from build123d import *

# Parameters (mm, degrees)
CROQUIS1_R              = 5.5
SALIENTE_EXTRUIR1_DEPTH = 10
CROQUIS3_W              = 5.5
CROQUIS3_H              = 15.5
SALIENTE_EXTRUIR2_DEPTH = 3


with BuildPart() as part:
    # Croquis1 → Saliente-Extruir1 (new body)
    with BuildSketch(Plane(origin=(0, 0, 0), x_dir=(1, 0, 0), z_dir=(0, 1, 0))):
        with Locations(Location((-6.881511077, -6.29378807, 0), (0, 0, 270))):
            Circle(CROQUIS1_R)
    extrude(amount=SALIENTE_EXTRUIR1_DEPTH)

    # Croquis3 → Saliente-Extruir2 (add)
    with BuildSketch(Plane(origin=(0, 0, 0), x_dir=(1, 0, 0), z_dir=(0, 1, 0))):
        with Locations((-6.881511077, -6.29378807)):
            Rectangle(CROQUIS3_W, CROQUIS3_H)
    extrude(amount=SALIENTE_EXTRUIR2_DEPTH)


solid = part.part
Verification items for the finished model (mm, model axes). A direction names the side the tool comes from. Give positions to 0.01 mm unless a question says otherwise; leave off trailing zeros. Order: outer loops, then holes, each group sorted by start corner. A loop starts at its lowest first (then second) coordinate and runs counter-clockwise, first axis right, second up. Notation, with made-up numbers: M -28,59.25 L -11,59.25 A27 ccw -11,82.25 Z; hole C -33,-24.75 d7. An arc over 180 degrees is marked long. Use one line per item in the form item = value. Start each with the question number.
Q1. Go/stop test with flat-tipped pins: pin 1 Ø4 at (y, z) = (9, 8.5) entering from -X; pin 2 Ø6 at (x, y) = (-10, 8.5) entering from +Z; pin 3 Ø0.9 at (y, z) = (1.5, -0.5) entering from +X. Record where each tip stops, or that it passes through.
Q2. Section check B-B (z = 0). Enter the section's corners in (x, y), then the cut area to 3 significant figures.
Q3. Scan lines: line 1 along Z through (x, y) = (-7, 4); line 2 along X through (y, z) = (2.5, 1.5); line 3 along Z through (x, y) = (-4, 0.5). Record each from-to range of solid material in increasing order. Write a range as [from, to].
Q4. Section check C-C (y = 4.25). Enter the section's corners in (x, z), then the cut area to 3 significant figures.
Q5. Access from +Z, -Z, +X, -X, +Y, -Y to the whole of each face (thin tool, end or side, straight path). Record for faces 1 (the flat face through (-4.132, 1, 13)), 2 (the flat face through (-4.132, 1, 0)), 3 (the cylindrical face through (-6.6, 4.9, 0.8)), 4 (the flat face through (-9.632, 1, 13)).
Q6. Section check A-A (x = -4.5). Enter the section's corners in (y, z), then the cut area to 3 significant figures.
Q7. Section check D-D (z = 11.25). Enter the section's corners in (x, y), then the cut area to 3 significant figures.
Evaluation:
q1.pin_1 = -12.38
q1.pin_2 = 11.79
q1.pin_3 = -4.13
q2.outline = M -9.63,0 L -4.13,0 L -4.13,3 L -9.63,3 Z
q2.area = 16.5 mm2
q3.line_1 = [0.8, 11.79]
q3.line_2 = [-9.63, -4.13]
q3.line_3 = [1.61, 10.98]
q4.outline = C -6.88,6.29 d11
q4.area = 95.0 mm2
q5.face_1 = +Z, +X, +Y, -Y
q5.face_2 = -Z, +X, +Y, -Y
q5.face_3 = +Y
q5.face_4 = +Z, -X, +Y, -Y
q6.outline = M 0,-1.46 L 3,-1.46 L 3,1.34 L 10,1.34 L 10,11.25 L 3,11.25 L 3,14.04 L 0,14.04 Z
q6.area = 116 mm2
q7.outline = M -9.63,0 L -4.13,0 L -4.13,3 L -4.5,3 L -4.5,10 L -9.27,10 L -9.27,3 L -9.63,3 Z
q7.area = 49.9 mm2
